CAD build for the part. Positions are in the model's coordinates, mm. Face numbers are marked on the shaded views. A direction names the side the tool comes from. Give positions to 0.01 mm unless a question says otherwise; leave off trailing zeros. Order: outer loops, then holes, each group sorted by start corner. A loop starts at its lowest first (then second) coordinate and runs counter-clockwise, first axis right, second up.
Item 1: Which spindle directions (+Z, -Z, +X, -X, +Y, -Y) get a long thin tool onto all of the face, cutting with end or side? Do the marked faces 1, 2 and 3. Say none if no direction does.
Item 2: Band-saw the part on D-D on y = -0.5. Give the cut face in (x, z) (3 decimals), plus the area to 3 significant figures.
Item 3: Band-saw the part on C-C on x = -12.5. Give the cut face in (y, z).
Item 4: Wall check: L1, parallel to Z at x = -32, y = 1; L2, parallel to X at y = -1, z = 1.25; L3, parallel to Z at x = -8, y = 0. Give the ranges that are in metal, low to high.
Item 5: Two-plate mould, pull along Z, no slides. Class the marked faces 4, 5 and 6: released by +Z, released by -Z, zero draft, split by the parting line, or undercut.
Item 6: Band-saw the part on B-B on z = 0. Give the cut face in (x, y).
Item 7: Band-saw the part on A-A on x = -5.5. Give the cut face in (y, z) (3 decimals).
Item 8: Flat gauge pins, fed straight in: P1, Ø1.5, axis at x = -3.5, z = -0.5, coming from the +Y side; P2, Ø2, axis at x = -17.5, y = 1, coming from the +Z side; P3, Ø1.9, axis at x = -6.5, y = 0, coming from the +Z side. Where does each tip first touch, or does it go through?
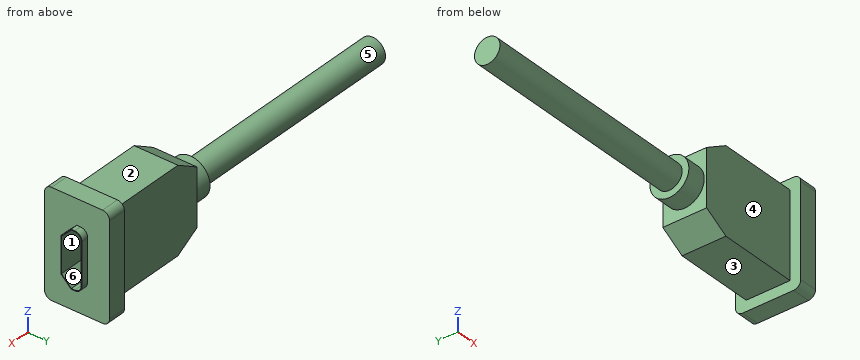
```python
from build123d import *

# Parameters (mm, degrees)
BOSS_EXTRUDE1_DEPTH = 3.1
SKETCH2_W           = 15
SKETCH2_H           = 9.2
BOSS_EXTRUDE2_DEPTH = 2.6
SKETCH3_R           = 2.75
BOSS_EXTRUDE3_DEPTH = 2.7
SKETCH4_R           = 1.8
BOSS_EXTRUDE4_DEPTH = 32
FILLET1_R           = 1
CUT_EXTRUDE1_DEPTH  = 7
BOSS_EXTRUDE5_DEPTH = 1


with BuildPart() as part:
    # Sketch1 → Boss-Extrude1 (new body, symmetric)
    with BuildSketch(Plane(origin=(0, 0, 0), x_dir=(1, 0, 0), z_dir=(0, 1, 0))):
        Polygon((0, 6), (0, -6), (-13.87, -6), (-17.25, -4), (-17.25, 4), (-13.87, 6), align=None)
    extrude(amount=BOSS_EXTRUDE1_DEPTH, both=True)

    # Sketch2 → Boss-Extrude2 (add)
    with BuildSketch(Plane(origin=(0, 0, 0), x_dir=(0, 0, -1), z_dir=(1, 0, 0))):
        Rectangle(SKETCH2_W, SKETCH2_H)
    extrude(amount=-BOSS_EXTRUDE2_DEPTH)

    # Sketch3 → Boss-Extrude3 (add)
    with BuildSketch(Plane.ZY.offset(17.25)):
        Circle(SKETCH3_R)
    extrude(amount=BOSS_EXTRUDE3_DEPTH)

    # Sketch4 → Boss-Extrude4 (add)
    with BuildSketch(Plane.ZY.offset(19.95)):
        Circle(SKETCH4_R)
    extrude(amount=BOSS_EXTRUDE4_DEPTH)

    # Fillet1
    fillet1_edges = [part.edges().sort_by_distance(p)[0] for p in [
        (-1.3, -4.6, 7.5),
        (-1.3, 4.6, 7.5),
        (-1.3, 4.6, -7.5),
        (-1.3, -4.6, -7.5),
    ]]
    fillet(fillet1_edges, radius=FILLET1_R)

    # Sketch5 → Cut-Extrude1 (cut)
    with BuildSketch(Plane(origin=(0, 0, 0), x_dir=(0, 0, -1), z_dir=(1, 0, 0))):
        with BuildLine():
            Line((2.975, 1.39), (-2.975, 1.39))
            ThreePointArc((-2.975, 1.39), (-3.611396103, 1.126396103), (-3.875, 0.49))
            Line((-3.875, 0.49), (-3.875, 0))
            Line((-3.875, 0), (-2.485, -1.39))
            Line((-2.485, -1.39), (2.485, -1.39))
            Line((2.485, -1.39), (3.875, 0))
            Line((3.875, 0), (3.875, 0.49))
            ThreePointArc((3.875, 0.49), (3.611396103, 1.126396103), (2.975, 1.39))
        make_face()
    extrude(amount=-CUT_EXTRUDE1_DEPTH, mode=Mode.SUBTRACT)

    # Sketch7 → Boss-Extrude5 (add)
    with BuildSketch(Plane(origin=(0, 0, 0), x_dir=(0, 0, -1), z_dir=(1, 0, 0))):
        with BuildLine():
            Line((2.975, 1.49), (-2.975, 1.49))
            ThreePointArc((-2.975, 1.49), (-3.682106781, 1.197106781), (-3.975, 0.49))
            Line((-3.975, 0.49), (-3.975, -0.041421356))
            Line((-3.975, -0.041421356), (-2.526421356, -1.49))
            Line((-2.526421356, -1.49), (2.526421356, -1.49))
            Line((2.526421356, -1.49), (3.975, -0.041421356))
            Line((3.975, -0.041421356), (3.975, 0.49))
            ThreePointArc((3.975, 0.49), (3.682106781, 1.197106781), (2.975, 1.49))
        make_face()
        with BuildLine():
            Line((-3.875, 0.49), (-3.875, 0))
            Line((-3.875, 0), (-2.485, -1.39))
            Line((-2.485, -1.39), (2.485, -1.39))
            Line((2.485, -1.39), (3.875, 0))
            Line((3.875, 0), (3.875, 0.49))
            ThreePointArc((3.875, 0.49), (3.611396103, 1.126396103), (2.975, 1.39))
            Line((2.975, 1.39), (-2.975, 1.39))
            ThreePointArc((-2.975, 1.39), (-3.611396103, 1.126396103), (-3.875, 0.49))
        make_face(mode=Mode.SUBTRACT)
    extrude(amount=BOSS_EXTRUDE5_DEPTH)


solid = part.part
```
The answers:
1. face 1: +X
1. face 2: +Z, -X, +Y, -Y
1. face 3: -Z, -X, +Y, -Y
2. outline: (-51.95, -1.729) - (-19.95, -1.729) - (-19.95, -2.704) - (-17.25, -2.704) - (-17.25, -4) - (-13.87, -6) - (-2.6, -6) - (-2.6, -7.5) - (0, -7.5) - (0, -3.516) - (1, -3.516) - (1, -3.375) - (-7, -3.375) - (-7, 3.375) - (1, 3.375) - (1, 3.516) - (0, 3.516) - (0, 7.5) - (-2.6, 7.5) - (-2.6, 6) - (-13.87, 6) - (-17.25, 4) - (-17.25, 2.704) - (-19.95, 2.704) - (-19.95, 1.729) - (-51.95, 1.729) - close
2. area: 286 mm2
3. outline: (-3.1, -6) - (3.1, -6) - (3.1, 6) - (-3.1, 6) - close
4. L1: z = -1.5 to 1.5
4. L2: x = -51.95 to -7
4. L3: z = -6 to 6
5. face 4: zero draft
5. face 5: split by the parting line
5. face 6: undercut
6. outline: (-51.95, -1.8) - (-19.95, -1.8) - (-19.95, -2.75) - (-17.25, -2.75) - (-17.25, -3.1) - (-2.6, -3.1) - (-2.6, -4.6) - (0, -4.6) - (0, -1.49) - (1, -1.49) - (1, -1.39) - (-7, -1.39) - (-7, 1.39) - (1, 1.39) - (1, 1.49) - (0, 1.49) - (0, 4.6) - (-2.6, 4.6) - (-2.6, 3.1) - (-17.25, 3.1) - (-17.25, 2.75) - (-19.95, 2.75) - (-19.95, 1.8) - (-51.95, 1.8) - close
7. outline: (-3.1, -6) - (3.1, -6) - (3.1, 6) - (-3.1, 6) - close; hole (-1.39, -2.485) - (0, -3.875) - (0.49, -3.875) arc R0.9 ccw to (1.39, -2.975) - (1.39, 2.975) arc R0.9 ccw to (0.49, 3.875) - (0, 3.875) - (-1.39, 2.485) - close
8. P1: stops at y = 3.1
8. P2: stops at z = 4.44
8. P3: stops at z = 6
